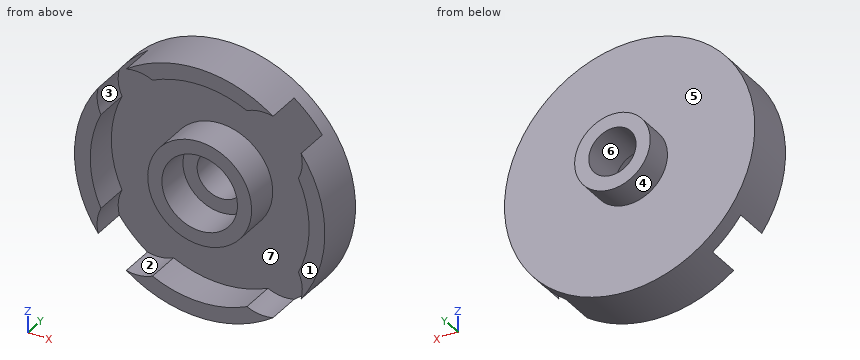
```python
from build123d import *

# Parameters (mm, degrees)
SKETCH1_R           = 7.95
BOSS_EXTRUDE1_DEPTH = 3.2
SKETCH2_R           = 2.4
BOSS_EXTRUDE2_DEPTH = 1.8
SHELL1_T            = -1
BOSS_EXTRUDE3_START = 2.2
SKETCH3_R           = 3.3
SKETCH3_R_2         = 2.4
BOSS_EXTRUDE3_DEPTH = 2.2
SKETCH4_R           = 2.45
CUT_EXTRUDE1_DEPTH  = 12.586414458
CIRPATTERN2_COUNT   = 4
SKETCH5_R           = 1.5
CUT_EXTRUDE2_DEPTH  = 13.304673909


with BuildPart() as part:
    # Sketch1 → Boss-Extrude1 (new body)
    with BuildSketch(Plane(origin=(0, 0, 0), x_dir=(1, 0, 0), z_dir=(0, 1, 0))):
        with Locations(Location((0, 0, 0), (0, 0, 270))):
            Circle(SKETCH1_R)
    extrude(amount=BOSS_EXTRUDE1_DEPTH)

    # Sketch2 → Boss-Extrude2 (add)
    with BuildSketch(Plane(origin=(0, 3.2, 0), x_dir=(1, 0, 0), z_dir=(0, 1, 0))):
        with Locations(Location((0, 0, 0), (0, 0, 270))):
            Circle(SKETCH2_R)
    extrude(amount=BOSS_EXTRUDE2_DEPTH)

    # Shell1
    shell1_openings = [part.faces().sort_by_distance(p)[0] for p in [
        (0, 0, 0),
    ]]
    offset(amount=SHELL1_T, openings=shell1_openings, kind=Kind.INTERSECTION)

    # Sketch3 → Boss-Extrude3 (add)
    with BuildSketch(Plane.XZ.offset(-2.2).offset(BOSS_EXTRUDE3_START)):
        with Locations(Location((0, 0, 0), (0, 0, 90))):
            Circle(SKETCH3_R)
        with Locations(Location((0, 0, 0), (0, 0, 90))):
            Circle(SKETCH3_R_2, mode=Mode.SUBTRACT)
    extrude(amount=-BOSS_EXTRUDE3_DEPTH)

    # Sketch4 → Cut-Extrude1 (cut, through all)
    with BuildSketch(Plane.XZ.offset(-2.2)):
        with Locations((-4.065863992, -4.065863992)):
            Circle(SKETCH4_R)
    cut_extrude1 = extrude(amount=CUT_EXTRUDE1_DEPTH, mode=Mode.SUBTRACT)

    # CirPattern2: Cut-Extrude1 ×4 about axis
    cirpattern2_axis = Axis((0, 0, 0), (0, 1, 0))
    for i in range(1, CIRPATTERN2_COUNT):
        add(cut_extrude1.rotate(cirpattern2_axis, i * 360 / CIRPATTERN2_COUNT), mode=Mode.SUBTRACT)

    # Sketch5 → Cut-Extrude2 (cut, through all)
    with BuildSketch(Plane(origin=(0, 5, 0), x_dir=(1, 0, 0), z_dir=(0, 1, 0))):
        with Locations(Location((0, 0, 0), (0, 0, 270))):
            Circle(SKETCH5_R)
    extrude(amount=-CUT_EXTRUDE2_DEPTH, mode=Mode.SUBTRACT)


solid = part.part
```
Geometry: final body of the model. Coordinates: model frame, mm. Face numbers are marked on the shaded views. A direction names the side the tool comes from. Round coordinates to 2 decimals unless told otherwise and drop trailing zeros. Order: outer loops, then holes, each group sorted by start corner. A loop starts at its lowest first (then second) coordinate and runs counter-clockwise, first axis right, second up. Notation, with made-up numbers: (15.25, -25) -> (56.25, -25) arc R10 cw to (56.25, -19) -> close; hole circle Ø3 at (-31, 89.25). An arc over 180 degrees is marked (long way). Use CSV: the item, a comma, the result in double quotes. Start each with the question number.
1) Draft query along Z for the marked faces 1, 2, 3 and 4. Return one class per face: +Z half, -Z half, draft (parallel to the pull), parting line (faces both ways), or undercut.
2) Section A-A (x = 0). Return the cut outline in (y, z), and give its area (3 significant figures).
3) Material intervals for line 1 along X through (y, z) = (1.2, 0); line 2 along Z through (x, y) = (-0.75, 0.65); line 3 along X through (y, z) = (4.15, 0), sorted ascending. Write a range as from..to.
4) Section B-B (z = 0). Return the cut outline in (x, y).
5) Section C-C (y = 0.85). Return the cut outline in (x, z), and give its area (3 significant figures).
6) First-contact query: pin 1 Ø2 at (y, z) = (1.5, -2) entering from +X; pin 2 Ø1 at (y, z) = (1.5, -5) entering from +X; pin 3 Ø1 at (x, y) = (-3.5, 2) entering from -Z. Flat tips, straight axial feed; report the tip coordinate or a pass-through.
7) Set-up query: the marked faces 5, 6 and 7. Return all of +Z, -Z, +X, -X, +Y, -Y with unobstructed straight access to the full face (end or side cutting, diameter ignored); none if empty.
8) Section D-D (y = 2.7). Return the cut outline in (x, z), and give its area (3 significant figures).
Returned:
1,face 1,"draft"
1,face 2,"undercut"
1,face 3,"undercut"
1,face 4,"parting line"
2,outline,"(0, -7.95) -> (3.2, -7.95) -> (3.2, -2.4) -> (5, -2.4) -> (5, -1.5) -> (2.2, -1.5) -> (2.2, -2.4) -> (0, -2.4) -> (0, -3.3) -> (2.2, -3.3) -> (2.2, -6.95) -> (0, -6.95) -> close; (0, 2.4) -> (2.2, 2.4) -> (2.2, 1.5) -> (5, 1.5) -> (5, 2.4) -> (3.2, 2.4) -> (3.2, 7.95) -> (0, 7.95) -> (0, 6.95) -> (2.2, 6.95) -> (2.2, 3.3) -> (0, 3.3) -> close"
2,area,"24.5 mm²"
3,line 1,"x = -7.95..-6.95, -3.3..-2.4, 2.4..3.3, 6.95..7.95"
3,line 2,"z = -7.91..-6.91, -3.21..-2.28, 2.28..3.21, 6.91..7.91"
3,line 3,"x = -2.4..-1.5, 1.5..2.4"
4,outline,"(-7.95, 0) -> (-6.95, 0) -> (-6.95, 2.2) -> (-3.3, 2.2) -> (-3.3, 0) -> (-2.4, 0) -> (-2.4, 2.2) -> (-1.5, 2.2) -> (-1.5, 5) -> (-2.4, 5) -> (-2.4, 3.2) -> (-7.95, 3.2) -> close; (1.5, 2.2) -> (2.4, 2.2) -> (2.4, 0) -> (3.3, 0) -> (3.3, 2.2) -> (6.95, 2.2) -> (6.95, 0) -> (7.95, 0) -> (7.95, 3.2) -> (2.4, 3.2) -> (2.4, 5) -> (1.5, 5) -> close"
5,outline,"(-6.44, -4.66) arc R2.45 cw to (-6.27, -3) arc R6.95 cw to (-6.27, 3) arc R2.45 cw to (-6.44, 4.66) arc R7.95 ccw to start; (-4.66, -6.44) arc R7.95 ccw to (4.66, -6.44) arc R2.45 cw to (3, -6.27) arc R6.95 cw to (-3, -6.27) arc R2.45 cw to start; (-4.66, 6.44) arc R2.45 cw to (-3, 6.27) arc R6.95 cw to (3, 6.27) arc R2.45 cw to (4.66, 6.44) arc R7.95 ccw to start; circle Ø6.6 at (0, 0); (6.27, -3) arc R2.45 cw to (6.44, -4.66) arc R7.95 ccw to (6.44, 4.66) arc R2.45 cw to (6.27, 3) arc R6.95 cw to start; hole circle Ø4.8 at (0, 0)"
5,area,"47.3 mm²"
6,pin 1,"stops at x = 7.89"
6,pin 2,"stops at x = 6.55"
6,pin 3,"stops at z = -7.36"
7,face 5,"+Y"
7,face 6,"+Y, -Y"
7,face 7,"-Y"
8,outline,"circle Ø15.9 at (0, 0); hole circle Ø3 at (0, 0)"
8,area,"191 mm²"
